Read the model definition and answer for the solid it produces. Units are mm, in the model's axes. A direction names the side the tool comes from. Give positions to 0.01 mm unless a question says otherwise; leave off trailing zeros. Order: outer loops, then holes, each group sorted by start corner. A loop starts at its lowest first (then second) coordinate and runs counter-clockwise, first axis right, second up.
Autodesk Inventor part; units mm, degrees
ref_plane "YZ Plane" through (0, 0, 0) normal (1, 0, 0) x (0, 1, 0)
ref_plane "XZ Plane" through (0, 0, 0) normal (0, 1, 0) x (-1, 0, 0)
ref_plane "XY Plane" through (0, 0, 0) normal (0, 0, 1) x (1, 0, 0)
sketch "スケッチ1" plane through (0, 0, 0) normal (0, 0, 1) x (1, 0, 0)
  line L0 (0, 0) -> (352, 0)
  line L1 (352, 0) -> (352, 5)
  line L2 (352, 5) -> (0, 5)
  line L3 (0, 5) -> (0, 0)
  line L4 (0, 0) -> (6, 0)
  line L5 (0, 1) -> (0, 0)
  dimension "d0" = 352
  dimension "d1" = 5
extrude "押し出し1" add sketch "スケッチ1" along normal blind 20
sketch "スケッチ3" plane through (0, 0, 0) normal (-1, 0, 0) x (0, 0, 1)
  line L0 (0, 5) -> (0, 0)
  line L1 (0, 0) -> (20, 0)
  line L2 (20, 5) -> (20, 0)
  line L3 (0, 5) -> (20, 5)
  circle A0 centre (4, 2.5) radius 1.2
  circle A1 centre (16, 2.5) radius 1.2
  dimension "d14" = 2.4
  dimension "d15" = 2.4
  dimension "d16" = 2.5
  dimension "d17" = 4
  dimension "d18" = 4
  dimension "d19" = 2.5
extrude "押し出し3" cut sketch "スケッチ3" against normal blind 3 contours A0 | A1
sketch "スケッチ4" plane through (0, 0, 0) normal (0, -1, 0) x (1, 0, 0)
  line L0 (0, 0) -> (352, 0)
  line L1 (352, 0) -> (352, 20)
  line L2 (0, 20) -> (352, 20)
  line L3 (0, 0) -> (0, 20)
  line L4 (2, 2) -> (350, 2)
  line L5 (350, 2) -> (350, 18)
  line L6 (350, 18) -> (2, 18)
  line L7 (2, 18) -> (2, 2)
  dimension "d22" = 2
  dimension "d23" = 2
  dimension "d24" = 2
  dimension "d25" = 2
extrude "押し出し4" cut sketch "スケッチ4" against normal blind 3 contours L7 L6 L5 L4
sketch "スケッチ5" plane through (0, 5, 0) normal (0, 1, 0) x (1, 0, 0)
  circle A0 centre (322, -10) radius 8
extrude "押し出し5" cut sketch "スケッチ5" against normal through all
sketch "スケッチ6" plane through (0, 5, 0) normal (0, 1, 0) x (1, 0, 0)
  circle A0 centre (340, -10) radius 3
extrude "押し出し6" cut sketch "スケッチ6" against normal through all
sketch "スケッチ7" plane through (0, 5, 0) normal (0, 1, 0) x (1, 0, 0)
  circle A0 centre (309.5, -10) radius 2
  circle A1 centre (288.5, -10) radius 3.5
  circle A2 centre (276.5, -10) radius 3.5
  circle A3 centre (309.5, -10) radius 4.5
  circle A4 centre (309.5, -10) radius 3.25
  circle A5 centre (309.5, -10) radius 3.5
extrude "押し出し7" cut sketch "スケッチ7" against normal through all contours A0 | A1 | A2 | A4 | A5
sketch "スケッチ8" plane through (352, 0, 0) normal (1, 0, 0) x (0, 0, -1)
  arc A0 (-17.0909, 3) -> (-14.9091, 3) centre (-16, 2.5) ccw
  arc A1 (-14.9091, 3) -> (-17.0909, 3) centre (-16, 2.5) ccw
  arc A2 (-2.9091, 3) -> (-5.0909, 3) centre (-4, 2.5) ccw
  arc A3 (-5.0909, 3) -> (-2.9091, 3) centre (-4, 2.5) ccw
extrude "押し出し8" cut sketch "スケッチ8" against normal blind 3
properties part number "arm1_L" material "アルミニウム 6061"
1) The part is cut by section C-C on x = 32.5. Determine the outline of the cut face in (y, z).
Final values:
outline: (0, 0) - (5, 0) - (5, 20) - (0, 20) - (0, 18) - (3, 18) - (3, 2) - (0, 2) - close
2) A tool of negligible diameter and unlimited length cuts with its end or side. For faces 3 (the face through (291.84, 4.01, 8.95)), 4 (the face through (336, 3, 10)), from which of +Z, -Z, +X, -X, +Y, -Y can it reach the whole face along a straight path? Write none if from no direction.
Final values:
face 3: +Y, -Y
face 4: -Y
3) Given pin 1 (1.9 mm diameter, centred on y = 2.5, z = 4, fed in from -X); pin 2 (1.4 mm diameter, centred on y = 2.5, z = 16, fed in from +X); pin 3 (1 mm diameter, centred on x = 150, z = 6.5, fed in from -Y), each flat-ended and moving along its own axis, determine where each tip first touches the part or whether it passes through.
Final values:
pin 1: stops at x = 3
pin 2: stops at x = 349
pin 3: stops at y = 3
4) For a pull along X with two mould halves and no side action, classify faces 1 (the face through (279.84, 4.01, 8.95)), 2 (the face through (175.2, 0, 1.8)) as released by +X, released by -X, zero draft, split by the parting line, or undercut.
Final values:
face 1: undercut
face 2: zero draft
5) Consider L1, parallel to X at y = 4.05, z = 10; L2, parallel to Z at x = 1.1, y = 2.5; L3, parallel to Z at x = 340, y = 4.1. Determine where each line is inside the solid, lowest interval first.
Final values:
L1: x = 0 to 273, 280 to 285, 292 to 306, 313 to 314, 330 to 337, 343 to 352
L2: z = 0 to 2.8, 5.2 to 14.8, 17.2 to 20
L3: z = 0 to 7, 13 to 20
6) The part is cut by section B-B on z = 10. Determine the outline of the cut face in (x, y).
Final values:
outline: (0, 0) - (2, 0) - (2, 3) - (273, 3) - (273, 5) - (0, 5) - close; (280, 3) - (285, 3) - (285, 5) - (280, 5) - close; (292, 3) - (306, 3) - (306, 5) - (292, 5) - close; (313, 3) - (314, 3) - (314, 5) - (313, 5) - close; (330, 3) - (337, 3) - (337, 5) - (330, 5) - close; (343, 3) - (350, 3) - (350, 0) - (352, 0) - (352, 5) - (343, 5) - close
7) The part is cut by section A-A on x = 340. Determine the outline of the cut face in (y, z), and give its area (3 significant figures).
Final values:
outline: (0, 0) - (5, 0) - (5, 7) - (3, 7) - (3, 2) - (0, 2) - close; (0, 18) - (3, 18) - (3, 13) - (5, 13) - (5, 20) - (0, 20) - close
area: 40.0 mm2
